Could you check a few things on this model? Use its own coordinates, in mm. Round coordinates to 2 decimals unless told otherwise and drop trailing zeros. Loops run counter-clockwise (first coordinate to the right, second up) from the corner with the lowest first, then second, coordinate; pieces in that order, holes last. Notation, with made-up numbers: (-32.75, 42.25) - (7.25, 42.25) arc R15 cw to (7.25, 54.25) - close; hole circle Ø5 at (-2, 63.25). An arc over 180 degrees is marked (long way). Use one line per item in the form item = value.
```python
from build123d import *

# Parameters (mm, degrees)
SKETCH1_W                                       = 100
SKETCH1_H                                       = 170
BOSS_EXTRUDE1_DEPTH                             = 3
CSK_FOR_M3_FLAT_HEAD_MACHINE_SCREW1_D           = 3.4
CSK_FOR_M3_FLAT_HEAD_MACHINE_SCREW1_DEPTH       = 7.5
CSK_FOR_M3_FLAT_HEAD_MACHINE_SCREW1_CSINK_D     = 6.3
CSK_FOR_M3_FLAT_HEAD_MACHINE_SCREW1_CSINK_ANGLE = 90
CSK_FOR_M3_FLAT_HEAD_MACHINE_SCREW1_TIP         = 1.021463052
FILLET1_R                                       = 5
CSK_FOR_M3_FLAT_HEAD_MACHINE_SCREW2_D           = 3.4
CSK_FOR_M3_FLAT_HEAD_MACHINE_SCREW2_DEPTH       = 7.5
CSK_FOR_M3_FLAT_HEAD_MACHINE_SCREW2_CSINK_D     = 6.3
CSK_FOR_M3_FLAT_HEAD_MACHINE_SCREW2_CSINK_ANGLE = 90
CSK_FOR_M3_FLAT_HEAD_MACHINE_SCREW2_TIP         = 1.021463052


with BuildPart() as part:
    # Sketch1 → Boss-Extrude1 (new body)
    with BuildSketch(Plane.XY):
        with Locations((50, 85)):
            Rectangle(SKETCH1_W, SKETCH1_H)
    extrude(amount=BOSS_EXTRUDE1_DEPTH)

    # CSK for M3 Flat Head Machine Screw1
    with Locations(Plane.XY.offset(3)):
        with Locations((5, 165), (95, 165), (95, 5), (5, 5)):
            CounterSinkHole(CSK_FOR_M3_FLAT_HEAD_MACHINE_SCREW1_D / 2, CSK_FOR_M3_FLAT_HEAD_MACHINE_SCREW1_CSINK_D / 2, depth=CSK_FOR_M3_FLAT_HEAD_MACHINE_SCREW1_DEPTH, counter_sink_angle=CSK_FOR_M3_FLAT_HEAD_MACHINE_SCREW1_CSINK_ANGLE)
            with Locations((0, 0, -(CSK_FOR_M3_FLAT_HEAD_MACHINE_SCREW1_DEPTH + CSK_FOR_M3_FLAT_HEAD_MACHINE_SCREW1_TIP / 2))):  # 118° drill point
                Cone(0, CSK_FOR_M3_FLAT_HEAD_MACHINE_SCREW1_D / 2, CSK_FOR_M3_FLAT_HEAD_MACHINE_SCREW1_TIP, mode=Mode.SUBTRACT)

    # Fillet1
    fillet1_edges = [part.edges().sort_by_distance(p)[0] for p in [
        (0, 170, 1.5),
        (100, 170, 1.5),
        (100, 0, 1.5),
        (0, 0, 1.5),
    ]]
    fillet(fillet1_edges, radius=FILLET1_R)

    # CSK for M3 Flat Head Machine Screw2
    with Locations(Plane(origin=(0, 0, 0), x_dir=(-1, 0, 0), z_dir=(0, 0, -1))):
        with Locations((-50, 135), (-50, 85), (-50, 35)):
            CounterSinkHole(CSK_FOR_M3_FLAT_HEAD_MACHINE_SCREW2_D / 2, CSK_FOR_M3_FLAT_HEAD_MACHINE_SCREW2_CSINK_D / 2, depth=CSK_FOR_M3_FLAT_HEAD_MACHINE_SCREW2_DEPTH, counter_sink_angle=CSK_FOR_M3_FLAT_HEAD_MACHINE_SCREW2_CSINK_ANGLE)
            with Locations((0, 0, -(CSK_FOR_M3_FLAT_HEAD_MACHINE_SCREW2_DEPTH + CSK_FOR_M3_FLAT_HEAD_MACHINE_SCREW2_TIP / 2))):  # 118° drill point
                Cone(0, CSK_FOR_M3_FLAT_HEAD_MACHINE_SCREW2_D / 2, CSK_FOR_M3_FLAT_HEAD_MACHINE_SCREW2_TIP, mode=Mode.SUBTRACT)


solid = part.part
```
1. For P1, Ø4.5, axis at x = 5, y = 5, coming from the +Z side; P2, Ø5.5, axis at x = 50, y = 35, coming from the -Z side; P3, Ø2, axis at x = 56, y = 62, coming from the -Z side; P4, Ø4, axis at x = 50, y = 85, coming from the -Z side, each with a flat end and sliding along its axis, tell me the tip position at first contact or that it passes through.
Solution:
P1 = 2.1
P2 = 0.4
P3 = 0
P4 = 1.15
2. If we section it at A-A, the plane y = 85: Write out the boundary of the cut face in (x, z), plus the area to 3 significant figures.
Solution:
outline = (0, 0) - (46.85, 0) - (48.3, 1.45) - (48.3, 3) - (0, 3) - close; (51.7, 1.45) - (53.15, 0) - (100, 0) - (100, 3) - (51.7, 3) - close
area = 288 mm^2
3. Please list where these lines run through material, in increasing order: line 1 along Y through (x, z) = (5, 1.2); line 2 along Y through (x, z) = (50, 1.8); line 3 along X through (y, z) = (5, 1.15).
Solution:
line_1 = 0 to 3.3, 6.7 to 163.3, 166.7 to 170
line_2 = 0 to 33.3, 36.7 to 83.3, 86.7 to 133.3, 136.7 to 170
line_3 = 0 to 3.3, 6.7 to 93.3, 96.7 to 100
4. We'd pull the mould along Y, two halves only. Please class faces 1 (the face through (0, 84, 1)), 2 (the face through (96.7, 5.07, 0.76)), 3 (the face through (99, 2, 2)), 4 (the face through (5.37, 163.34, 0.76)): +Y half, -Y half, draft (parallel to the pull), parting line (faces both ways), or undercut.
Solution:
face_1 = draft
face_2 = undercut
face_3 = -Y half
face_4 = undercut
